Check sheet for the modelled part. Datum: model origin and axes. Units: mm. A direction names the side the tool comes from. Round coordinates to 2 decimals unless told otherwise and drop trailing zeros. Write each loop counter-clockwise with the first axis right and the second up, starting at its lowest first coordinate (ties: lowest second). Pieces come first, ordered by that corner, then holes. Notation, with made-up numbers: (51.25, 19.5) -> (84.25, 19.5) arc R21 ccw to (84.25, 54.5) -> close; hole circle Ø10 at (-27.5, -29). An arc over 180 degrees is marked (long way). One line per item, written item: value. Start each with the question number.
```python
from build123d import *

# Parameters (mm, degrees)
F5_W      = 7.9
F5_H      = 0.9
F5_W_2    = 3.6
F5_H_2    = 4.8
F5_W_3    = 13.7
F6_DEPTH  = 6.775
F7_DEPTH  = 12
F10_DEPTH = 2.15
F11_D     = 8.8
F8_R      = 5.975
F8_R_2    = 4.3
F12_DEPTH = 8.5


with BuildPart() as f6:
    # F5 (on Top) → F6 (new body)
    with BuildSketch(Plane.XY):
        with Locations((-6.85, 4.7)):
            Rectangle(F5_W, F5_H)
        with Locations((9, -0.75)):
            Rectangle(F5_W_2, F5_H_2)
        Polygon((-10.8, 4.25), (-10.8, -4.25), (10.8, -4.25), (10.8, -3.15), (7.2, -3.15), (7.2, 1.65), (10.8, 1.65), (10.8, 4.25), (-2.9, 4.25), align=None)
        with Locations((3.95, 4.7)):
            Rectangle(F5_W_3, F5_H)
    extrude(amount=F6_DEPTH)

    # F5 (on Top) → F7 (join)
    with BuildSketch(Plane.XY):
        with Locations((3.95, 4.7)):
            Rectangle(F5_W_3, F5_H)
        with Locations((9, -0.75)):
            Rectangle(F5_W_2, F5_H_2)
    extrude(amount=-F7_DEPTH)

    # F9 (on face) → F10 (join)
    with BuildSketch(Plane(origin=(0, 0, 0), x_dir=(1, 0, 0), z_dir=(0, 0, -1))):
        Polygon((3.95, 4.25), (3.95, -4.25), (10.8, -4.25), (10.8, -1.65), (7.2, -1.65), (7.2, 3.15), (10.8, 3.15), (10.8, 4.25), align=None)
    extrude(amount=F10_DEPTH)

    # F11 (through all)
    with Locations(Plane(origin=(0, 5.15, 0), x_dir=(-1, 0, 0), z_dir=(0, 1, 0))):
        with Locations((-3.9, 0)):
            Hole(F11_D / 2)

    # F8 (on face) → F12 (join)
    with BuildSketch(Plane(origin=(0, 5.15, 0), x_dir=(-1, 0, 0), z_dir=(0, 1, 0))):
        Polygon((10.8, 6.775), (-10.8, 6.775), (-10.8, -12), (2.9, -12), (2.9, 0), (10.8, 0), align=None)
        with Locations((-3.9, 0)):
            Circle(F8_R, mode=Mode.SUBTRACT)
        with Locations((-3.9, 0)):
            Circle(F8_R)
        with Locations((-3.9, 0)):
            Circle(F8_R_2, mode=Mode.SUBTRACT)
    extrude(amount=F12_DEPTH)


solid = f6.part
```
1. Cross-section at C-C (z = -5.75). Record the cut outline in (x, y).
2. Cross-section at D-D (y = -2). Record the cut outline in (x, z) (3 decimals).
3. Depth check by flat-ended pin: pin 1 Ø3.5 at (x, z) = (4.5, -3.5) entering from -Y; pin 2 Ø2 at (x, z) = (5.5, 2) entering from +Y; pin 3 Ø4.5 at (y, z) = (11, -5.5) entering from -X; pin 4 Ø1.1 at (x, z) = (8.5, -8.5) entering from -Y. Enter the tip coordinate at first touch or a pass-through.
4. Cross-section at B-B (y = 6.75). Record the cut outline in (x, z) (3 decimals).
5. Release check for a two-part mould opening along Z. For faces 4 (the face through (0.2, 13.65, -2.5)), 5 (the face through (3.327, 0.384, 4.363)), 6 (the face through (9, -4, -2.15)) record: +Z half, -Z half, draft (parallel to the pull), parting line (faces both ways), or undercut.
6. Access from +Z, -Z, +X, -X, +Y, -Y to the whole of each face (thin tool, end or side, straight path). Record for faces 1 (the face through (-2.9, 9, -6)), 2 (the face through (9, 1.65, -7)), 3 (the face through (7.2, -1, -7)).
7. Material ranges on probe 1 along Y at (x, z) = (9, -8.25); probe 2 along Z at (x, y) = (3.9, 1.25) (3 decimals); probe 3 along X at (y, z) = (-3, -3.25), recorded low to high.
8. Cross-section at A-A (x = 3.9). Record the cut outline in (y, z) (3 decimals).
Working result:
1. outline: (-2.9, 4.25) -> (10.8, 4.25) -> (10.8, 13.65) -> (-2.9, 13.65) -> close; (7.2, -3.15) -> (10.8, -3.15) -> (10.8, 1.65) -> (7.2, 1.65) -> close
2. outline: (-10.8, 0) -> (-0.5, 0) arc R4.4 cw (long way) to (7.2, -2.91) -> (7.2, -12) -> (10.8, -12) -> (10.8, 6.775) -> (-10.8, 6.775) -> close
3. pin 1: stops at y = 4.25
3. pin 2: passes through
3. pin 3: stops at x = -2.9
3. pin 4: stops at y = -3.15
4. outline: (-10.8, 0) -> (-2.9, 0) -> (-2.9, -12) -> (10.8, -12) -> (10.8, 6.775) -> (-10.8, 6.775) -> close; hole circle Ø8.6 at (3.9, 0)
5. face 4: draft
5. face 5: undercut
5. face 6: -Z half
6. face 1: -Z, -X, +Y, -Y
6. face 2: -Z, +X, -X
6. face 3: -Z, -X, -Y
7. probe 1: y = -3.15 to 1.65, 4.25 to 13.65
7. probe 2: z = 4.4 to 6.775
7. probe 3: x = 7.2 to 10.8
8. outline: (-4.25, 4.4) -> (5.15, 4.4) -> (5.15, 4.3) -> (13.65, 4.3) -> (13.65, 6.775) -> (-4.25, 6.775) -> close; (4.25, -12) -> (13.65, -12) -> (13.65, -4.3) -> (5.15, -4.3) -> (5.15, -4.4) -> (4.25, -4.4) -> close
